Input: part model. Units: mm. Frame: model coordinates. A direction names the side the tool comes from. Round coordinates to 2 decimals unless told otherwise and drop trailing zeros. Order: outer loops, then holes, each group sorted by start corner. A loop starts at its lowest first (then second) coordinate and runs counter-clockwise, first axis right, second up.
Item 1: Cut plane B-B on z = 0. Output: boundary loops of the cut face in (x, y), then the cut area to 3 significant figures.
Item 2: Reachability of faces 1 (the flat face through (-5, 0, -1.7)), 2 (the cylindrical face through (9.92, -0.03, 2.65)), 3 (the flat face through (10, -1.85, 0)) from +Z, -Z, +X, -X, +Y, -Y: full face, straight path, thin tool, end or side. Return the list, or none.
Item 3: First-contact query: pin 1 (1 mm diameter, centred on x = 1.5, y = 1, fed in from -Z); pin 2 (3 mm diameter, centred on x = 12.5, z = 0, fed in from -Y); pin 3 (1.3 mm diameter, centred on y = -0.5, z = 0, fed in from -X). Flat tips, straight axial feed; report the tip coordinate or a pass-through.
Item 4: Mould query, pull axis Z, two halves, no side actions, for faces 4 (the flat face through (0, 0, 0)), 5 (the flat face through (10, 1.85, 0)), 6 (the cylindrical face through (-3.158, -1.231, -3.595)), 7 (the cylindrical face through (9.92, 0.03, -2.65)). Classes: released by +Z, released by -Z, zero draft, split by the parting line, or undercut.
Item 5: Cut plane A-A on y = 0. Output: boundary loops of the cut face in (x, z), then the cut area to 3 significant figures.
Item 6: Line query: L1, parallel to Y at x = -6, z = 0; L2, parallel to Z at x = -5.75, y = 0; L3, parallel to X at y = -0.75, z = 1. Output: solid intervals per line, ascending.
```python
from build123d import *

# Parameters (mm, degrees)
SALIENTE_EXTRUIR1_DEPTH      = 16
SALIENTE_EXTRUIR2_DEPTH      = 2
SALIENTE_EXTRUIR2_DEPTH_BACK = 9
CROQUIS2_R                   = 3.8
SALIENTE_EXTRUIR3_DEPTH      = 2
CHAFL_N1_SIZE                = 2


with BuildPart() as part:
    # Croquis1 → Saliente-Extruir1 (new body)
    with BuildSketch(Plane(origin=(0, 0, 0), x_dir=(0, 0, -1), z_dir=(1, 0, 0))):
        with BuildLine():
            Line((-1.897366596, 1.85), (1.897366596, 1.85))
            ThreePointArc((1.897366596, 1.85), (2.65, 0), (1.897366596, -1.85))
            Line((1.897366596, -1.85), (-1.897366596, -1.85))
            ThreePointArc((-1.897366596, -1.85), (-2.65, 0), (-1.897366596, 1.85))
        make_face()
    extrude(amount=SALIENTE_EXTRUIR1_DEPTH)

    # Croquis2 → Saliente-Extruir2 (add, two sides: drawn at the far end of the back side and taken through both)
    with BuildSketch(Plane(origin=(0, 0, 0), x_dir=(0, 0, -1), z_dir=(1, 0, 0)).offset(-SALIENTE_EXTRUIR2_DEPTH_BACK)):
        Circle(CROQUIS2_R)
        with BuildLine():
            Line((1.7, 1.549193338), (1.7, -1.549193338))
            ThreePointArc((1.7, -1.549193338), (-2.3, 0), (1.7, 1.549193338))
        make_face(mode=Mode.SUBTRACT)
    extrude(amount=SALIENTE_EXTRUIR2_DEPTH + SALIENTE_EXTRUIR2_DEPTH_BACK)

    # Croquis3 → Saliente-Extruir3 (add)
    with BuildSketch(Plane(origin=(0, 0, 0), x_dir=(0, 0, -1), z_dir=(1, 0, 0))):
        with BuildLine():
            Line((-1.897366596, 1.85), (1.897366596, 1.85))
            ThreePointArc((1.897366596, 1.85), (0, 2.65), (-1.897366596, 1.85))
        make_face()
        with BuildLine():
            Line((-1.897366596, -1.85), (1.897366596, -1.85))
            ThreePointArc((1.897366596, -1.85), (0, -2.65), (-1.897366596, -1.85))
        make_face()
    extrude(amount=SALIENTE_EXTRUIR3_DEPTH)

    # Chaflán1
    # the kernel refuses this chamfer: 2 mm, written as the material it adds along each edge
    with BuildSketch(Plane(origin=(2, 0, 0), x_dir=(0, 0.4143114997605186, 0.91013514445174), z_dir=(0, -0.91013514445174, 0.4143114997605186))) as chafl_n1_piece_1_section:
        Polygon((2.65, -CHAFL_N1_SIZE), (2.65 + CHAFL_N1_SIZE, 0), (2.65, 0), align=None)
    chafl_n1_piece_1 = revolve(axis=Axis((2, 0, 0), (-1, 0, 0)), revolution_arc=311.048068347, mode=Mode.PRIVATE)
    chafl_n1_piece_1 = split(chafl_n1_piece_1, bisect_by=Plane(origin=(2, 1.85, 0), z_dir=(0, -1, 0)), keep=Keep.TOP, mode=Mode.PRIVATE)
    chafl_n1_piece_1 = split(chafl_n1_piece_1, bisect_by=Plane(origin=(2, -1.85, 0), z_dir=(0, 1, 0)), keep=Keep.TOP, mode=Mode.PRIVATE)
    chafl_n1_piece_1 = chafl_n1_piece_1 & Plane(origin=(2, 0, 0), x_dir=(0, 0, -1), z_dir=(-1, 0, 0)) * Cylinder(3.8, 19, mode=Mode.PRIVATE)
    add(chafl_n1_piece_1)
    with BuildSketch(Plane(origin=(2, -1.85, -7.040732572), x_dir=(1, 0, 0), z_dir=(0, 0, 1))) as chafl_n1_piece_2_section:
        Polygon((CHAFL_N1_SIZE, 0), (0, -CHAFL_N1_SIZE), (0, 0), align=None)
    chafl_n1_piece_2 = extrude(amount=14.081465144, mode=Mode.PRIVATE)
    chafl_n1_piece_2 = chafl_n1_piece_2 & Plane(origin=(2, 0, 0), x_dir=(0, 0.6981132075471701, -0.7159873947551046), z_dir=(-1, 0, 0)) * Cylinder(2.65, 37, mode=Mode.PRIVATE)
    add(chafl_n1_piece_2)
    with BuildSketch(Plane(origin=(2, 0, 0), x_dir=(0, -0.4143114997605186, -0.91013514445174), z_dir=(0, 0.91013514445174, -0.4143114997605186))) as chafl_n1_piece_3_section:
        Polygon((2.65, -CHAFL_N1_SIZE), (2.65 + CHAFL_N1_SIZE, 0), (2.65, 0), align=None)
    chafl_n1_piece_3 = revolve(axis=Axis((2, 0, 0), (-1, 0, 0)), revolution_arc=311.048068347, mode=Mode.PRIVATE)
    chafl_n1_piece_3 = split(chafl_n1_piece_3, bisect_by=Plane(origin=(2, 1.85, 0), z_dir=(0, -1, 0)), keep=Keep.TOP, mode=Mode.PRIVATE)
    chafl_n1_piece_3 = split(chafl_n1_piece_3, bisect_by=Plane(origin=(2, -1.85, 0), z_dir=(0, 1, 0)), keep=Keep.TOP, mode=Mode.PRIVATE)
    chafl_n1_piece_3 = chafl_n1_piece_3 & Plane(origin=(2, 0, 0), x_dir=(0, 0, -1), z_dir=(-1, 0, 0)) * Cylinder(3.8, 19, mode=Mode.PRIVATE)
    add(chafl_n1_piece_3)
    with BuildSketch(Plane(origin=(2, 1.85, -7.040732572), x_dir=(1, 0, 0), z_dir=(0, 0, 1))) as chafl_n1_piece_4_section:
        Polygon((CHAFL_N1_SIZE, 0), (0, CHAFL_N1_SIZE), (0, 0), align=None)
    chafl_n1_piece_4 = extrude(amount=14.081465144, mode=Mode.PRIVATE)
    chafl_n1_piece_4 = chafl_n1_piece_4 & Plane(origin=(2, 0, 0), x_dir=(0, -0.6981132075471701, 0.7159873947551046), z_dir=(-1, 0, 0)) * Cylinder(2.65, 37, mode=Mode.PRIVATE)
    add(chafl_n1_piece_4)
    with BuildSketch(Plane(origin=(2, 1.85, -7.040732572), x_dir=(1, 0, 0), z_dir=(0, 0, 1))) as chafl_n1_piece_5a_section:
        Polygon((CHAFL_N1_SIZE, 0), (0, CHAFL_N1_SIZE), (0, 0), align=None)
    chafl_n1_piece_5a = extrude(amount=14.081465144, mode=Mode.PRIVATE)
    chafl_n1_piece_5a = chafl_n1_piece_5a - Plane(origin=(2, 0, 0), x_dir=(0, -0.6981132075471701, 0.7159873947551046), z_dir=(-1, 0, 0)) * Cylinder(2.65, 37, mode=Mode.PRIVATE)
    chafl_n1_piece_5a = chafl_n1_piece_5a & Plane(origin=(2, 0, 0), x_dir=(0, 0, -1), z_dir=(-1, 0, 0)) * Cylinder(3.8, 37, mode=Mode.PRIVATE)
    with BuildSketch(Plane(origin=(2, 0, 0), x_dir=(0, 0.4143114997605186, 0.91013514445174), z_dir=(0, -0.91013514445174, 0.4143114997605186))) as chafl_n1_piece_5b_section:
        Polygon((2.65, -CHAFL_N1_SIZE), (2.65 + CHAFL_N1_SIZE, 0), (2.65, 0), align=None)
    chafl_n1_piece_5b = revolve(axis=Axis((2, 0, 0), (-1, 0, 0)), revolution_arc=311.048068347, mode=Mode.PRIVATE)
    chafl_n1_piece_5b = split(chafl_n1_piece_5b, bisect_by=Plane(origin=(2, 1.85, 0), z_dir=(0, 1, 0)), keep=Keep.TOP, mode=Mode.PRIVATE)
    chafl_n1_piece_5b = chafl_n1_piece_5b & Plane(origin=(2, 0, 0), x_dir=(0, 0, -1), z_dir=(-1, 0, 0)) * Cylinder(3.8, 19, mode=Mode.PRIVATE)
    chafl_n1_piece_5 = chafl_n1_piece_5a & chafl_n1_piece_5b
    add(chafl_n1_piece_5)
    with BuildSketch(Plane(origin=(2, 0, 0), x_dir=(0, 0.4143114997605186, 0.91013514445174), z_dir=(0, -0.91013514445174, 0.4143114997605186))) as chafl_n1_piece_6a_section:
        Polygon((2.65, -CHAFL_N1_SIZE), (2.65 + CHAFL_N1_SIZE, 0), (2.65, 0), align=None)
    chafl_n1_piece_6a = revolve(axis=Axis((2, 0, 0), (-1, 0, 0)), revolution_arc=311.048068347, mode=Mode.PRIVATE)
    chafl_n1_piece_6a = split(chafl_n1_piece_6a, bisect_by=Plane(origin=(2, -1.85, 0), z_dir=(0, -1, 0)), keep=Keep.TOP, mode=Mode.PRIVATE)
    chafl_n1_piece_6a = chafl_n1_piece_6a & Plane(origin=(2, 0, 0), x_dir=(0, 0, -1), z_dir=(-1, 0, 0)) * Cylinder(3.8, 19, mode=Mode.PRIVATE)
    with BuildSketch(Plane(origin=(2, -1.85, -7.040732572), x_dir=(1, 0, 0), z_dir=(0, 0, 1))) as chafl_n1_piece_6b_section:
        Polygon((CHAFL_N1_SIZE, 0), (0, -CHAFL_N1_SIZE), (0, 0), align=None)
    chafl_n1_piece_6b = extrude(amount=14.081465144, mode=Mode.PRIVATE)
    chafl_n1_piece_6b = chafl_n1_piece_6b - Plane(origin=(2, 0, 0), x_dir=(0, 0.6981132075471701, -0.7159873947551046), z_dir=(-1, 0, 0)) * Cylinder(2.65, 37, mode=Mode.PRIVATE)
    chafl_n1_piece_6b = chafl_n1_piece_6b & Plane(origin=(2, 0, 0), x_dir=(0, 0, -1), z_dir=(-1, 0, 0)) * Cylinder(3.8, 37, mode=Mode.PRIVATE)
    chafl_n1_piece_6 = chafl_n1_piece_6a & chafl_n1_piece_6b
    add(chafl_n1_piece_6)
    with BuildSketch(Plane(origin=(2, -1.85, -7.040732572), x_dir=(1, 0, 0), z_dir=(0, 0, 1))) as chafl_n1_piece_7a_section:
        Polygon((CHAFL_N1_SIZE, 0), (0, -CHAFL_N1_SIZE), (0, 0), align=None)
    chafl_n1_piece_7a = extrude(amount=14.081465144, mode=Mode.PRIVATE)
    chafl_n1_piece_7a = chafl_n1_piece_7a - Plane(origin=(2, 0, 0), x_dir=(0, 0.6981132075471701, -0.7159873947551046), z_dir=(-1, 0, 0)) * Cylinder(2.65, 37, mode=Mode.PRIVATE)
    chafl_n1_piece_7a = chafl_n1_piece_7a & Plane(origin=(2, 0, 0), x_dir=(0, 0, -1), z_dir=(-1, 0, 0)) * Cylinder(3.8, 37, mode=Mode.PRIVATE)
    with BuildSketch(Plane(origin=(2, 0, 0), x_dir=(0, -0.4143114997605186, -0.91013514445174), z_dir=(0, 0.91013514445174, -0.4143114997605186))) as chafl_n1_piece_7b_section:
        Polygon((2.65, -CHAFL_N1_SIZE), (2.65 + CHAFL_N1_SIZE, 0), (2.65, 0), align=None)
    chafl_n1_piece_7b = revolve(axis=Axis((2, 0, 0), (-1, 0, 0)), revolution_arc=311.048068347, mode=Mode.PRIVATE)
    chafl_n1_piece_7b = split(chafl_n1_piece_7b, bisect_by=Plane(origin=(2, -1.85, 0), z_dir=(0, -1, 0)), keep=Keep.TOP, mode=Mode.PRIVATE)
    chafl_n1_piece_7b = chafl_n1_piece_7b & Plane(origin=(2, 0, 0), x_dir=(0, 0, -1), z_dir=(-1, 0, 0)) * Cylinder(3.8, 19, mode=Mode.PRIVATE)
    chafl_n1_piece_7 = chafl_n1_piece_7a & chafl_n1_piece_7b
    add(chafl_n1_piece_7)
    with BuildSketch(Plane(origin=(2, 1.85, -7.040732572), x_dir=(1, 0, 0), z_dir=(0, 0, 1))) as chafl_n1_piece_8a_section:
        Polygon((CHAFL_N1_SIZE, 0), (0, CHAFL_N1_SIZE), (0, 0), align=None)
    chafl_n1_piece_8a = extrude(amount=14.081465144, mode=Mode.PRIVATE)
    chafl_n1_piece_8a = chafl_n1_piece_8a - Plane(origin=(2, 0, 0), x_dir=(0, -0.6981132075471701, 0.7159873947551046), z_dir=(-1, 0, 0)) * Cylinder(2.65, 37, mode=Mode.PRIVATE)
    chafl_n1_piece_8a = chafl_n1_piece_8a & Plane(origin=(2, 0, 0), x_dir=(0, 0, -1), z_dir=(-1, 0, 0)) * Cylinder(3.8, 37, mode=Mode.PRIVATE)
    with BuildSketch(Plane(origin=(2, 0, 0), x_dir=(0, -0.4143114997605186, -0.91013514445174), z_dir=(0, 0.91013514445174, -0.4143114997605186))) as chafl_n1_piece_8b_section:
        Polygon((2.65, -CHAFL_N1_SIZE), (2.65 + CHAFL_N1_SIZE, 0), (2.65, 0), align=None)
    chafl_n1_piece_8b = revolve(axis=Axis((2, 0, 0), (-1, 0, 0)), revolution_arc=311.048068347, mode=Mode.PRIVATE)
    chafl_n1_piece_8b = split(chafl_n1_piece_8b, bisect_by=Plane(origin=(2, 1.85, 0), z_dir=(0, 1, 0)), keep=Keep.TOP, mode=Mode.PRIVATE)
    chafl_n1_piece_8b = chafl_n1_piece_8b & Plane(origin=(2, 0, 0), x_dir=(0, 0, -1), z_dir=(-1, 0, 0)) * Cylinder(3.8, 19, mode=Mode.PRIVATE)
    chafl_n1_piece_8 = chafl_n1_piece_8a & chafl_n1_piece_8b
    add(chafl_n1_piece_8)

    # Chaflán2: read off the stored shape, not the designer's step
    # Chaflán2 outline → Chaflán2 (revolve)
    with BuildSketch(Plane.YX):
        Polygon((2.3, 0), (1.3, 0), (2.3, -1), align=None)
    revolve(axis=Axis((0, 0, 0), (1, 0, 0)))


solid = part.part
```
From the geometry:
1. outline: (-9, -3.8) - (2.05, -3.8) - (4, -1.85) - (16, -1.85) - (16, 1.85) - (4, 1.85) - (2.05, 3.8) - (-9, 3.8) - (-9, 2.3) - (-1, 2.3) - (0, 1.3) - (0, -1.3) - (-1, -2.3) - (-9, -2.3) - close
1. area: 99.0 mm2
2. face 1: -X
2. face 2: +Z, +X
2. face 3: +Z, -Z, +X, -Y
3. pin 1: stops at z = -3.77
3. pin 2: stops at y = -1.85
3. pin 3: stops at x = 0
4. face 4: undercut
4. face 5: zero draft
4. face 6: split by the parting line
4. face 7: released by -Z
5. outline: (-9, -3.8) - (2.85, -3.8) - (4, -2.65) - (16, -2.65) - (16, 2.65) - (4, 2.65) - (2.85, 3.8) - (-9, 3.8) - (-9, 2.3) - (-1, 2.3) - (0, 1.3) - (0, -1.3) - (-0.4, -1.7) - (-9, -1.7) - close
5. area: 126 mm2
6. L1: y = -3.8 to -2.3, 2.3 to 3.8
6. L2: z = -3.8 to -1.7, 2.3 to 3.8
6. L3: x = 0 to 16
